Check sheet for the modelled part. Datum: model origin and axes. Units: mm. Round coordinates to 2 decimals unless told otherwise and drop trailing zeros. Write each loop counter-clockwise with the first axis right and the second up, starting at its lowest first coordinate (ties: lowest second). Pieces come first, ordered by that corner, then holes. Notation, with made-up numbers: (-29, -23.75) -> (1, -23.75) arc R14 cw to (1, -8.75) -> close; hole circle Ø11 at (-36.5, 1.5). An arc over 180 degrees is marked (long way). One line per item, written item: value.
from build123d import *

# Parameters (mm, degrees)
BOSS_EXTRUDE1_DEPTH     = 30
SKETCH2_W               = 8.32
SKETCH2_H               = 8.5
SKETCH2_H_2             = 10.4
SKETCH2_W_2             = 4.158973904
SKETCH2_H_3             = 8.284744262
CUT_EXTRUDE5_DEPTH      = 8.32
CUT_EXTRUDE5_DEPTH_BACK = 8.32


with BuildPart() as part:
    # Sketch1 → Boss-Extrude1 (new body)
    with BuildSketch(Plane.XY):
        with BuildLine():
            Line((-61.072637036, 102.678177008), (-71.843049169, 72.656622079))
            ThreePointArc((-71.843049169, 72.656622079), (-38.845852098, 94.547390677), (0, 102.229873289))
            Line((0, 102.229873289), (0, 122.669843323))
            ThreePointArc((0, 122.669843323), (-24.83617604, 119.381808628), (-48.25837108, 110.490937356))
            ThreePointArc((-48.25837108, 110.490937356), (-54.800605836, 106.806147253), (-61.072637036, 102.678177008))
        make_face()
        with BuildLine():
            ThreePointArc((0, 137.710014326), (-25.468170629, 126.474444633), (-48.25837108, 110.490937356))
            ThreePointArc((-48.25837108, 110.490937356), (-24.83617604, 119.381808628), (0, 122.669843323))
            Line((0, 122.669843323), (0, 125.181241323))
            ThreePointArc((0, 125.181241323), (-5.008687502, 130.189928825), (0, 135.198616327))
            Line((0, 135.198616327), (0, 137.710014326))
        make_face()
    extrude(amount=BOSS_EXTRUDE1_DEPTH)

    # Sketch2 → Cut-Extrude5 (cut, two sides)
    with BuildSketch(Plane.XY.offset(15)) as cut_extrude5_sk:
        with Locations((-16.418701703, 104.318970145)):
            Rectangle(SKETCH2_W, SKETCH2_H)
        with Locations((-24.923280466, 103.197968007)):
            Rectangle(SKETCH2_W, SKETCH2_H_2)
        with Locations((-2.079486952, 106.272425537)):
            Rectangle(SKETCH2_W_2, SKETCH2_H_3)
    extrude(amount=CUT_EXTRUDE5_DEPTH, mode=Mode.SUBTRACT)
    extrude(cut_extrude5_sk.sketch, amount=-CUT_EXTRUDE5_DEPTH_BACK, mode=Mode.SUBTRACT)

    # Mirror3: part across plane


with BuildPart() as part_1:
    add(part.part)
    add(part.part.mirror(Plane(origin=(0, 0, 30), x_dir=(0, 0, 1), z_dir=(-1, 0, 0))))


solid = part_1.part
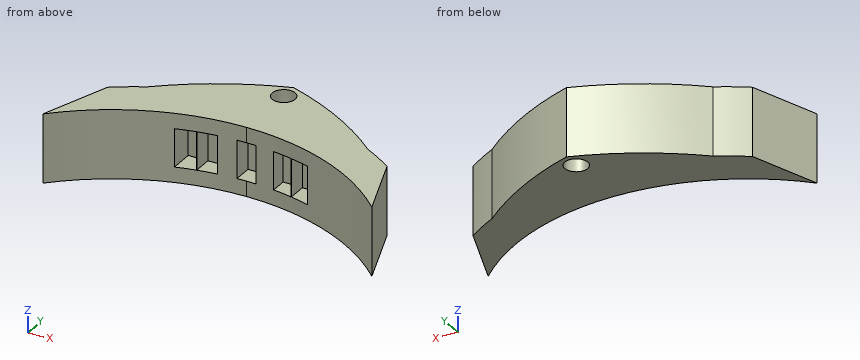
Item 1: Thickness scan on line 1 (X direction, y = 101, z = 11.75); line 2 (Y direction, x = 0, z = 11.75); line 3 (X direction, y = 84.5, z = 8.5). Record the ranges inside material, lowest first.
Answer:
line 1: x = -61.67 to -29.08, -20.76 to -20.58, 20.58 to 20.76, 29.08 to 61.67
line 2: y = 110.41 to 125.18, 135.2 to 137.71
line 3: x = -67.59 to -57.48, 57.48 to 67.59
Item 2: Sectioned sample at A-A on z = 18. Enter the section's corners in (x, y), and give its area (3 significant figures).
Answer:
outline: (-71.84, 72.66) arc R102.05 cw to (-29.08, 98) -> (-29.08, 108.4) -> (-20.76, 108.4) -> (-20.76, 100.1) arc R102.05 cw to (-20.58, 100.13) -> (-20.58, 108.57) -> (-12.26, 108.57) -> (-12.26, 101.49) arc R102.05 cw to (-4.16, 102.15) -> (-4.16, 110.41) -> (4.16, 110.41) -> (4.16, 102.15) arc R102.05 cw to (12.26, 101.49) -> (12.26, 108.57) -> (20.58, 108.57) -> (20.58, 100.13) arc R102.05 cw to (20.76, 100.1) -> (20.76, 108.4) -> (29.08, 108.4) -> (29.08, 98) arc R102.05 cw to (71.84, 72.66) -> (61.07, 102.68) arc R108.62 ccw to (48.26, 110.49) arc R142.15 ccw to (0, 137.71) arc R142.15 ccw to (-48.26, 110.49) arc R108.62 ccw to (-61.07, 102.68) -> close; hole circle Ø10.02 at (0, 130.19)
area: 3,010 mm^2
Item 3: Sectioned sample at B-B on x = -24.5. Enter the section's corners in (y, z).
Answer:
outline: (99.25, 0) -> (127.02, 0) -> (127.02, 30) -> (99.25, 30) -> (99.25, 23.32) -> (108.4, 23.32) -> (108.4, 6.68) -> (99.25, 6.68) -> close
Item 4: Sectioned sample at D-D on x = 8.5. Enter the section's corners in (y, z).
Answer:
outline: (101.88, 0) -> (134.61, 0) -> (134.61, 30) -> (101.88, 30) -> close
Item 5: Sectioned sample at C-C on y = 120.5. Enter the section's corners in (x, z), and give its area (3 significant figures).
Answer:
outline: (-35.14, 0) -> (35.14, 0) -> (35.14, 30) -> (-35.14, 30) -> close
area: 2,110 mm^2
Item 6: Depth check by flat-ended pin: P1, Ø9, axis at x = -1.5, y = 104.5, coming from the -Z side; P2, Ø9, axis at y = 106, z = 11.5, coming from the -X side; P3, Ø9.5, axis at y = 104.5, z = 16.5, coming from the +X side; P4, Ø2.5, axis at y = 104.5, z = 14, coming from the +X side. Enter the tip coordinate at first touch or a pass-through.
Answer:
P1: stops at z = 0
P2: stops at x = -61.5
P3: stops at x = 62.12
P4: stops at x = 60.26
